Check sheet for the modelled part. Datum: model origin and axes. Units: mm. Give positions to 0.01 mm unless a question says otherwise; leave off trailing zeros. Order: outer loops, then holes, each group sorted by start corner. A loop starts at its lowest first (then second) coordinate and runs counter-clockwise, first axis right, second up.
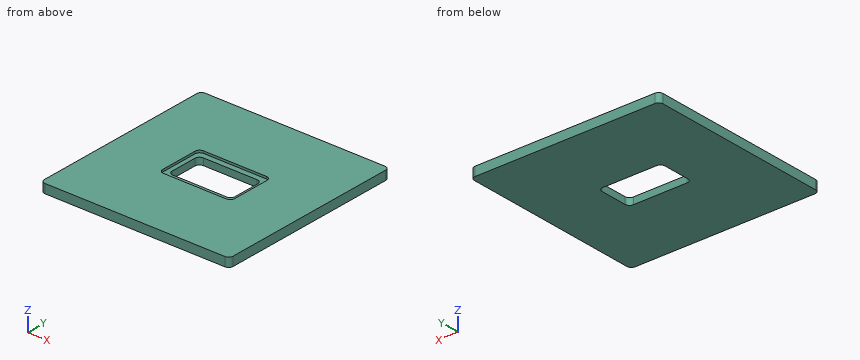
```python
from build123d import *

# Parameters (mm, degrees)
F1_DEPTH = 12.7
F3_DEPTH = 3.175


with BuildPart() as f1:
    # F0 (on Top) → F1 (new body)
    with BuildSketch(Plane.XY):
        with BuildLine():
            Line((213.760845, 133.35), (-40.239155, 133.35))
            ThreePointArc((-40.239155, 133.35), (-44.729283, 131.490128), (-46.589155, 127))
            Line((-46.589155, 127), (-46.589155, -127))
            ThreePointArc((-46.589155, -127), (-44.729283, -131.490128), (-40.239155, -133.35))
            Line((-40.239155, -133.35), (213.760845, -133.35))
            ThreePointArc((213.760845, -133.35), (218.250973, -131.490128), (220.110845, -127))
            Line((220.110845, -127), (220.110845, 127))
            ThreePointArc((220.110845, 127), (218.250973, 131.490128), (213.760845, 133.35))
        make_face()
        with BuildLine():
            ThreePointArc((42.310845, 19.05), (44.170717, 23.540128), (48.660845, 25.4))
            Line((48.660845, 25.4), (124.860845, 25.4))
            ThreePointArc((124.860845, 25.4), (129.350973, 23.540128), (131.210845, 19.05))
            Line((131.210845, 19.05), (131.210845, -19.05))
            ThreePointArc((131.210845, -19.05), (129.350973, -23.540128), (124.860845, -25.4))
            Line((124.860845, -25.4), (48.660845, -25.4))
            ThreePointArc((48.660845, -25.4), (44.170717, -23.540128), (42.310845, -19.05))
            Line((42.310845, -19.05), (42.310845, 19.05))
        make_face(mode=Mode.SUBTRACT)
    extrude(amount=F1_DEPTH)

    # F2 (on face) → F3 (cut)
    with BuildSketch(Plane.XY.offset(12.7)):
        with BuildLine():
            Line((131.20583, 33.17691), (42.30583, 33.17691))
            ThreePointArc((42.30583, 33.17691), (37.815701, 31.317038), (35.95583, 26.82691))
            Line((35.95583, 26.82691), (35.95583, -27.14809))
            ThreePointArc((35.95583, -27.14809), (37.815701, -31.638218), (42.30583, -33.49809))
            Line((42.30583, -33.49809), (131.20583, -33.49809))
            ThreePointArc((131.20583, -33.49809), (135.695958, -31.638218), (137.55583, -27.14809))
            Line((137.55583, -27.14809), (137.55583, 26.82691))
            ThreePointArc((137.55583, 26.82691), (135.695958, 31.317038), (131.20583, 33.17691))
        make_face()
        with BuildLine():
            Line((124.860845, -25.4), (48.660845, -25.4))
            ThreePointArc((48.660845, -25.4), (44.170717, -23.540128), (42.310845, -19.05))
            Line((42.310845, -19.05), (42.310845, 19.05))
            ThreePointArc((42.310845, 19.05), (44.170717, 23.540128), (48.660845, 25.4))
            Line((48.660845, 25.4), (124.860845, 25.4))
            ThreePointArc((124.860845, 25.4), (129.350973, 23.540128), (131.210845, 19.05))
            Line((131.210845, 19.05), (131.210845, -19.05))
            ThreePointArc((131.210845, -19.05), (129.350973, -23.540128), (124.860845, -25.4))
        make_face(mode=Mode.SUBTRACT)
    extrude(amount=-F3_DEPTH, mode=Mode.SUBTRACT)


solid = f1.part
```
Q1. Material ranges on line 1 (Y direction, x = 104.5, z = 9); line 2 (X direction, y = 12, z = 1.5); line 3 (X direction, y = -13.5, z = 11.25), recorded low to high.
Q2. Sectioned sample at B-B, the plane z = 3.75. Record the cut outline in (x, y).
Q3. Sectioned sample at A-A, the plane x = 94.5. Record the cut outline in (y, z) (3 decimals).
Q4. Sectioned sample at C-C, the plane y = 30. Record the cut outline in (x, z) (3 decimals), plus the area to 3 significant figures.
Filled in:
1. line 1: y = -133.35 to -25.4, 25.4 to 133.35
1. line 2: x = -46.59 to 42.31, 131.21 to 220.11
1. line 3: x = -46.59 to 35.96, 137.56 to 220.11
2. outline: (-46.59, -127) arc R6.35 ccw to (-40.24, -133.35) - (213.76, -133.35) arc R6.35 ccw to (220.11, -127) - (220.11, 127) arc R6.35 ccw to (213.76, 133.35) - (-40.24, 133.35) arc R6.35 ccw to (-46.59, 127) - close; hole (42.31, -19.05) arc R6.35 ccw to (48.66, -25.4) - (124.86, -25.4) arc R6.35 ccw to (131.21, -19.05) - (131.21, 19.05) arc R6.35 ccw to (124.86, 25.4) - (48.66, 25.4) arc R6.35 ccw to (42.31, 19.05) - close
3. outline: (-133.35, 0) - (-25.4, 0) - (-25.4, 9.525) - (-33.498, 9.525) - (-33.498, 12.7) - (-133.35, 12.7) - close; (25.4, 0) - (133.35, 0) - (133.35, 12.7) - (33.177, 12.7) - (33.177, 9.525) - (25.4, 9.525) - close
4. outline: (-46.589, 0) - (220.111, 0) - (220.111, 12.7) - (136.706, 12.7) - (136.706, 9.525) - (36.805, 9.525) - (36.805, 12.7) - (-46.589, 12.7) - close
4. area: 3,070 mm2
